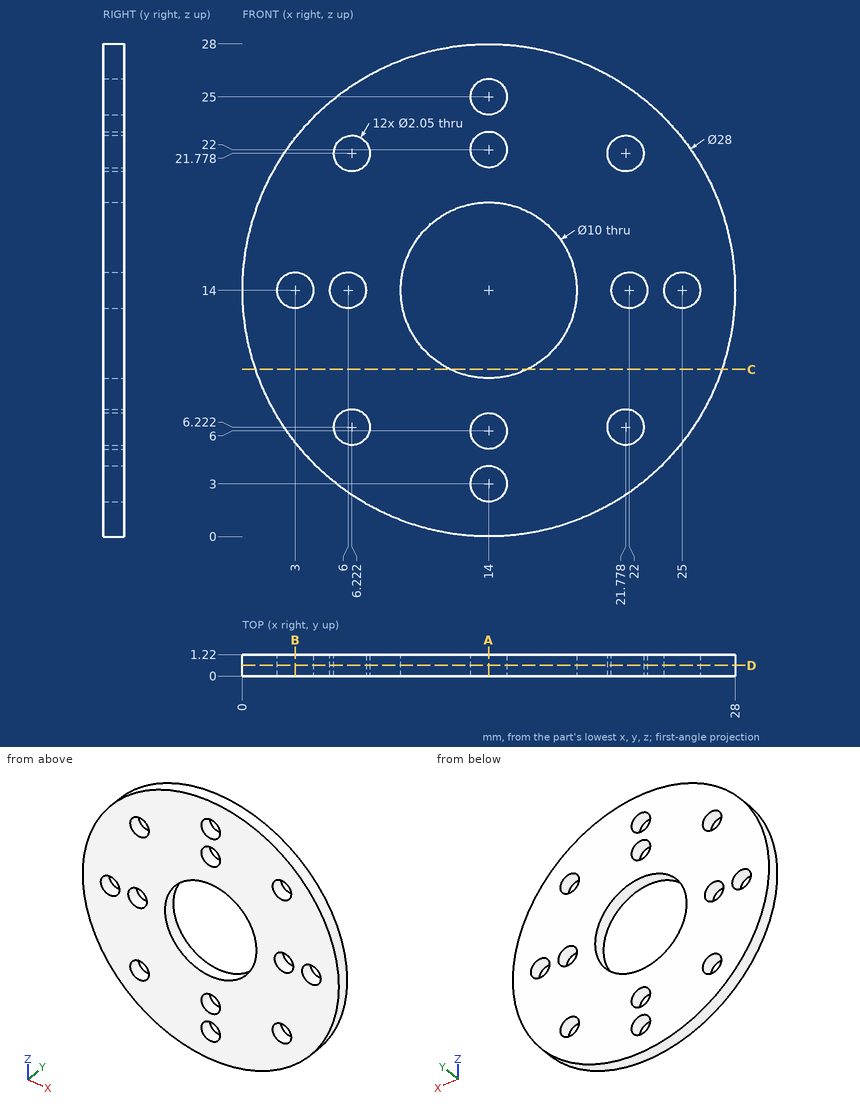
Input: dimensioned drawing with shaded views. Units: mm. Origin: part minimum x, y, z. Give positions to 0.01 mm unless a question says otherwise; leave off trailing zeros. Write each loop counter-clockwise with the first axis right and the second up, starting at its lowest first coordinate (ties: lowest second). Pieces come first, ordered by that corner, then holes.
1. First-contact query: pin 1 (1.6 mm diameter, centred on x = 14, z = 25, fed in from -Y). Flat tip, straight axial feed; report the tip coordinate or a pass-through.
2. Section query A-A (x = 14). Return the cut outline in (y, z) (3 decimals).
3. Material intervals for line 1 along Z through (x, y) = (14, 0.65) (3 decimals); line 2 along X through (y, z) = (0.35, 22) (1 decimal), sorted ascending.
4. Section query D-D (y = 0.6). Count the separate pieces of the cut face and the enclosed holes in it, then the cut area to 3 significant figures.
5. Section query B-B (x = 3). Return the cut outline in (y, z) (1 decimal), then the cut area to 3 significant figures.
6. Section query C-C (z = 9.5). Return the cut outline in (x, y), then the cut area to 3 significant figures.
Output values:
1. pin 1: passes through
2. outline: (0, 0) - (1.22, 0) - (1.22, 1.975) - (0, 1.975) - close; (0, 4.025) - (1.22, 4.025) - (1.22, 4.975) - (0, 4.975) - close; (0, 7.025) - (1.22, 7.025) - (1.22, 9) - (0, 9) - close; (0, 19) - (1.22, 19) - (1.22, 20.975) - (0, 20.975) - close; (0, 23.025) - (1.22, 23.025) - (1.22, 23.975) - (0, 23.975) - close; (0, 26.025) - (1.22, 26.025) - (1.22, 28) - (0, 28) - close
3. line 1: z = 0 to 1.975, 4.025 to 4.975, 7.025 to 9, 19 to 20.975, 23.025 to 23.975, 26.025 to 28
3. line 2: x = 2.5 to 5.2, 7.2 to 13, 15 to 20.8, 22.8 to 25.5
4. separate pieces: 1
4. enclosed holes: 13
4. area: 498 mm2
5. outline: (0, 5.3) - (1.2, 5.3) - (1.2, 13) - (0, 13) - close; (0, 15) - (1.2, 15) - (1.2, 22.7) - (0, 22.7) - close
5. area: 18.6 mm2
6. outline: (0.74, 0) - (11.82, 0) - (11.82, 1.22) - (0.74, 1.22) - close; (16.18, 0) - (27.26, 0) - (27.26, 1.22) - (16.18, 1.22) - close
6. area: 27.0 mm2
